Input: dimensioned drawing with shaded views. Units: mm. Origin: part minimum x, y, z. Round coordinates to 2 decimals unless told otherwise and drop trailing zeros. Loops run counter-clockwise (first coordinate to the right, second up) from the corner with the lowest first, then second, coordinate; pieces in that order, holes last. Notation, with made-up numbers: (76, -7.75) -> (115, -7.75) arc R21 ccw to (115, 23.25) -> close; hole circle Ø8 at (9.25, 9.25). An arc over 180 degrees is marked (long way). Answer as a JSON object with one key per item and string values.
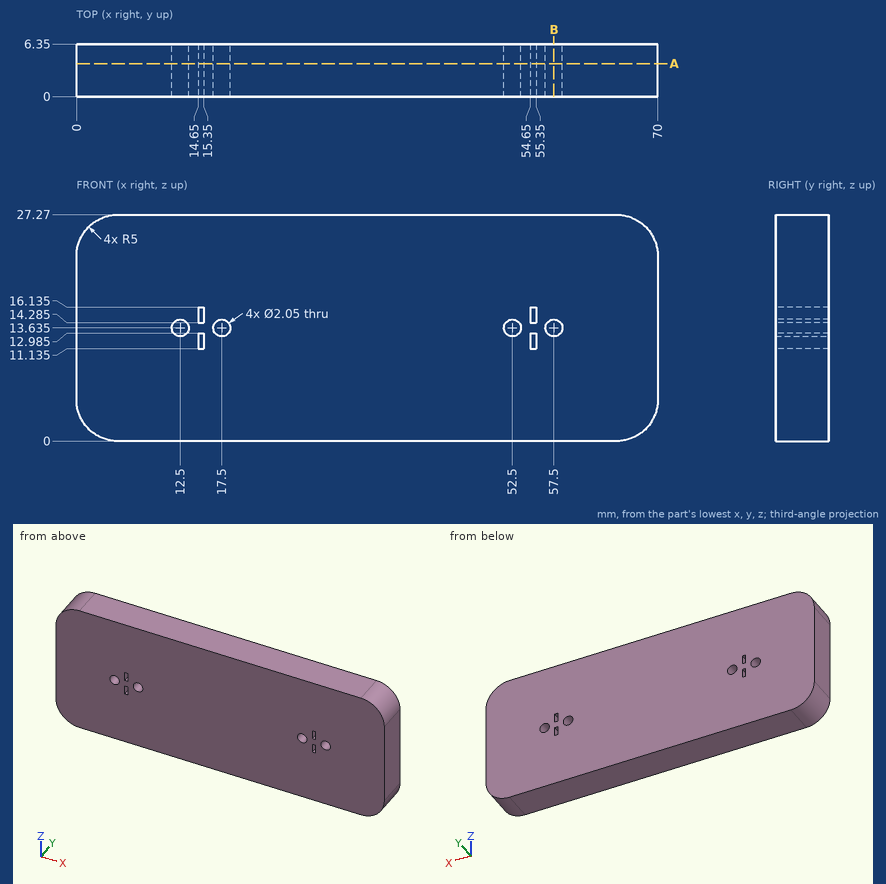
1) Contact query for flat-ended pins moving along their axis: P1, Ø1.2, axis at x = 12.5, z = 13.635, coming from the +Y side; P2, Ø3.5, axis at x = 57.5, z = 13.635, coming from the -Y side. Output: stop coordinate, or through.
Output:
{"P1": "passes through", "P2": "stops at y = 0"}
2) Section B-B, the plane x = 57.5. Output: boundary loops of the cut face in (y, z), plus the area to 3 significant figures.
Output:
{"outline": "(0, 0) -> (6.35, 0) -> (6.35, 12.61) -> (0, 12.61) -> close; (0, 14.66) -> (6.35, 14.66) -> (6.35, 27.27) -> (0, 27.27) -> close", "area": "160 mm^2"}
3) Ray query, probe 1 along Z at (x, y) = (15, 3.5) (3 decimals); probe 2 along X at (y, z) = (4.25, 12.25); probe 3 along X at (y, z) = (3, 14). Return the intervals inside material, ascending.
Output:
{"probe 1": "z = 0 to 11.135, 12.985 to 14.285, 16.135 to 27.27", "probe 2": "x = 0 to 14.65, 15.35 to 54.65, 55.35 to 70", "probe 3": "x = 0 to 11.54, 13.46 to 16.54, 18.46 to 51.54, 53.46 to 56.54, 58.46 to 70"}
4) Section A-A, the plane y = 4. Count the separate pieces of the cut face and the enclosed holes in it, plus the area to 3 significant figures.
Output:
{"separate pieces": "1", "enclosed holes": "8", "area": "1,870 mm^2"}
